Autodesk Inventor part; units mm, degrees
ref_plane "YZ Plane" through (0, 0, 0) normal (1, 0, 0) x (0, 1, 0)
ref_plane "XZ Plane" through (0, 0, 0) normal (0, 1, 0) x (-1, 0, 0)
ref_plane "XY Plane" through (0, 0, 0) normal (0, 0, 1) x (1, 0, 0)
sketch "Эскиз1" plane through (0, 0, 0) normal (0, 0, 1) x (1, 0, 0)
  circle A0 centre (0.9164, -10.9801) radius 1.6008
  arc A1 (-10.5243, 2.5819) -> (-10.0836, 1.5104) centre (-11.5836, 1.5199) ccw
  arc A2 (12.3571, 0.4579) -> (11.9164, 1.5294) centre (13.4164, 1.5199) ccw
  circle A3 centre (-11.5836, 1.5199) radius 1.5
  circle A4 centre (13.4164, 1.5199) radius 1.5
  line L0 (-21.9797, -65.2227) -> (23.8125, -65.2227)
  line L1 (23.8125, -65.2227) -> (23.8125, 68.2625)
  line L2 (23.8125, 68.2625) -> (-21.9797, 68.2625)
  line L3 (-21.9797, 68.2625) -> (-21.9797, -65.2227)
  line L4 (-21.9797, -65.2227) -> (23.8125, 68.2625) construction
  line L5 (23.8125, -65.2227) -> (-21.9797, 68.2625) construction
  point P0 (0, 0)
  point P1 (-10.0836, 1.5104)
  point P2 (12.3571, 0.4579)
  point P3 (11.9164, 1.5294)
extrude "Выдавливание1" add sketch "Эскиз1" along normal blind 3
sketch "Эскиз2" plane through (0, 0, 3) normal (0, 0, 1) x (1, 0, 0)
  line L0 (23.8125, -65.2227) -> (23.8125, 68.2625)
  line L1 (23.8125, 68.2625) -> (-21.9797, 68.2625)
  line L2 (-21.9797, 68.2625) -> (-21.9797, -65.2227)
  line L3 (-21.9797, -65.2227) -> (23.8125, -65.2227)
  circle A0 centre (-11.5836, 1.5199) radius 1.5
  circle A1 centre (13.4164, 1.5199) radius 1.5
  circle A2 centre (0.9164, -10.9801) radius 1.6008
  line L4 (-11.5836, 1.5199) -> (13.4164, 1.5199)
  line L5 (0.9164, 14.0199) -> (0.9164, -10.9801)
  circle A3 centre (0.9164, 1.5199) radius 4
  point P0 (0, 0)
  dimension "d2" = 8
extrude "Выдавливание2" cut sketch "Эскиз2" against normal blind 3 contours A3 L5 L4 | L4 L5 A3 | L5 A3 L4 | L4 A3 L5
sketch "Эскиз3" plane through (0, 0, 3) normal (0, 0, 1) x (1, 0, 0)
  circle A0 centre (0.9164, 1.5199) radius 4
  line L0 (23.8125, -65.2227) -> (23.8125, 68.2625)
  line L1 (23.8125, 68.2625) -> (-21.9797, 68.2625)
  line L2 (-21.9797, 68.2625) -> (-21.9797, -65.2227)
  line L3 (-21.9797, -65.2227) -> (23.8125, -65.2227)
  circle A1 centre (-11.5836, 1.5199) radius 1.5
  circle A2 centre (13.4164, 1.5199) radius 1.5
  circle A3 centre (0.9164, -10.9801) radius 1.6008
  line L4 (0.9164, 1.5199) -> (0.9164, 18.5199)
  circle A4 centre (0.9164, 18.5199) radius 3
  point P0 (0, 0)
  dimension "d5" = 17
  dimension "d6" = 6
extrude "Выдавливание3" add sketch "Эскиз3" along normal blind 8 contours A4
sketch "Эскиз4" plane through (0, 0, 3) normal (0, 0, 1) x (1, 0, 0)
  circle A0 centre (0.9164, 18.5199) radius 3
  circle A1 centre (0.9164, 43.7699) radius 9.5
  circle A2 centre (0.9164, 43.7699) radius 13.15
  circle A3 centre (0.9164, 18.5199) radius 3
  circle A4 centre (0.9164, 1.5199) radius 4
  line L0 (23.8125, -65.2227) -> (23.8125, 68.2625)
  line L1 (23.8125, 68.2625) -> (-21.9797, 68.2625)
  line L2 (-21.9797, 68.2625) -> (-21.9797, -65.2227)
  line L3 (-21.9797, -65.2227) -> (23.8125, -65.2227)
  circle A5 centre (-11.5836, 1.5199) radius 1.5
  circle A6 centre (13.4164, 1.5199) radius 1.5
  circle A7 centre (0.9164, -10.9801) radius 1.6008
  point P0 (0, 0)
  dimension "d17" = 42.25
  dimension "d18" = 0
extrude "Выдавливание4" add sketch "Эскиз4" along normal blind 6 contours A2
sketch "Эскиз5" plane through (0, 0, 3) normal (0, 0, 1) x (1, 0, 0)
  circle A0 centre (0.9164, -10.9801) radius 1.6008
  circle A1 centre (13.4164, 1.5199) radius 1.5
  circle A2 centre (-11.5836, 1.5199) radius 1.5
  line L0 (23.8125, -65.2227) -> (23.8125, 68.2625)
  line L1 (23.8125, 68.2625) -> (-21.9797, 68.2625)
  line L2 (-21.9797, 68.2625) -> (-21.9797, -65.2227)
  line L3 (-21.9797, -65.2227) -> (23.8125, -65.2227)
  circle A3 centre (0.9164, 43.7699) radius 13.15
  circle A4 centre (0.9164, 1.5199) radius 4
  circle A5 centre (0.9164, 43.7699) radius 3
  point P0 (0, 0)
  dimension "d12" = 6
  dimension "d16" = 0
extrude "Выдавливание5" cut sketch "Эскиз5" against normal blind 8 contours A5
sketch "Эскиз6" plane through (0.9164, 43.7699, 3) normal (0, 0, 1) x (1, 0, 0)
  circle A0 centre (0, 0) radius 7.5
  circle A1 centre (0, 0) radius 13.15
  circle A2 centre (0, 0) radius 9.5
  point P0 (-0.9164, -43.7699)
  dimension "d19" = 15
extrude "Выдавливание6" cut sketch "Эскиз6" against normal blind 1 contours A0
ref_plane "РабПлоскость1" through (0, 0, -6) normal (0, 0, -1) x (-1, 0, 0)
sketch "Эскиз7" plane through (0, 0, -6) normal (0, 0, -1) x (-1, 0, 0)
  circle A0 centre (-0.9164, 43.7699) radius 13.15
  circle A1 centre (-0.9164, 43.7699) radius 9.5
  point P0 (0, 0)
extrude "Выдавливание7" add sketch "Эскиз7" against normal blind 6
sketch "Эскиз8" plane through (0.9164, 43.7699, 9) normal (0, 0, 1) x (1, 0, 0)
  circle A0 centre (0, 0) radius 13.15
  circle A1 centre (0, 0) radius 9.5
  point P0 (-0.9164, -43.7699)
extrude "Выдавливание8" cut sketch "Эскиз8" against normal blind 6
sketch "Эскиз9" plane through (0.9164, 43.7699, -6) normal (0, 0, -1) x (-1, 0, 0)
  circle A0 centre (0, 0) radius 13.15
  point P0 (0.9164, -43.7699)
extrude "Выдавливание9" add sketch "Эскиз9" against normal blind 3
sketch "Эскиз10" plane through (0.9164, 43.7699, -3) normal (0, 0, 1) x (1, 0, 0)
  circle A0 centre (0, 0) radius 3
  circle A1 centre (0, 0) radius 7.5
  point P0 (-0.9164, -43.7699)
extrude "Выдавливание10" cut sketch "Эскиз10" against normal blind 1
sketch "Эскиз12" plane through (0, 0, 3) normal (0, 0, 1) x (1, 0, 0)
  circle A0 centre (0.9164, 18.5199) radius 3
  circle A1 centre (0.9164, 1.5199) radius 4
  line L0 (23.8125, -65.2227) -> (23.8125, 68.2625)
  line L1 (23.8125, 68.2625) -> (-21.9797, 68.2625)
  line L2 (-21.9797, 68.2625) -> (-21.9797, -65.2227)
  line L3 (-21.9797, -65.2227) -> (23.8125, -65.2227)
  circle A2 centre (-11.5836, 1.5199) radius 1.5
  circle A3 centre (13.4164, 1.5199) radius 1.5
  circle A4 centre (0.9164, -10.9801) radius 1.6008
  circle A5 centre (0.9164, 43.7699) radius 7.5
  circle A6 centre (0.9164, 43.7699) radius 9.5
  point P0 (0, 0)
  dimension "d33" = 19
extrude "Выдавливание12" cut sketch "Эскиз12" against normal blind 6 contours A5 | A6
sketch "Эскиз13" plane through (0.9164, 43.7699, -3) normal (0, 0, 1) x (1, 0, 0)
  circle A0 centre (0, 0) radius 3
  point P0 (-0.9164, -43.7699)
extrude "Выдавливание13" cut sketch "Эскиз13" against normal through all
properties part number "пластина для редуктора"
Could you check a few things on this model? Use its own coordinates, in mm. A direction names the side the tool comes from. Coordinates: 2 decimals unless noted, no trailing zeros. Write each loop counter-clockwise with the first axis right and the second up, starting at its lowest first coordinate (ties: lowest second). Pieces come first, ordered by that corner, then holes. Notation, with made-up numbers: M 64.5,-36.5 L 87.5,-36.5 A24 cw 87.5,-18.5 Z; hole C 60,85 d11. An arc over 180 degrees is marked long. One line per question, with ' | ' between items.
1) Imagine slicing it at B-B, the plane x = 19. Write out the boundary of the cut face in (y, z), and give its area (3 significant figures).
Checks:
outline: M -65.22,0 L 68.26,0 L 68.26,3 L -65.22,3 Z | area: 400 mm²
2) Imagine slicing it at C-C, the plane z = -1.25. Write out the boundary of the cut face in (x, y), and give its area (3 significant figures).
Checks:
outline: C 0.92,43.77 d26.3; hole C 0.92,43.77 d19 | area: 260 mm²
3) Imagine slicing it at A-A, the plane x = 0.5. Give the number of separate pieces and of enclosed holes in the cut face, and give its area (3 significant figures).
Checks:
separate pieces: 4 | enclosed holes: 0 | area: 432 mm²
4) If we mould it in two halves opening along Y, with no side actions, what happens to faces 1 (the face through (0.708, -12.567, 1.479)), 2 (the face through (1, 68.262, 1)), 3 (the face through (6, 2, 0))? For each: released by +Y, released by -Y, zero draft, split by the parting line, or undercut.
Checks:
face 1: undercut | face 2: released by +Y | face 3: zero draft
5) Imagine slicing it at D-D, the plane y = 54.5. Write out the boundary of the cut face in (x, z).
Checks:
outline: M -21.98,0 L -6.69,0 L -6.69,-6 L 8.52,-6 L 8.52,0 L 23.81,0 L 23.81,3 L -21.98,3 Z
6) For pin 1 Ø5 at (x, y) = (0.92, -10.98) entering from +Z; pin 2 Ø9.5 at (x, y) = (4, 41) entering from +Z; pin 3 Ø3.5 at (x, y) = (-11.58, 1.52) entering from -Z; pin 4 Ø24 at (x, y) = (0.92, 43.77) entering from -Z, each with a flat end and sliding along its axis, tell me the tip position at first contact or that it passes through.
Checks:
pin 1: z = 3 | pin 2: z = -3 | pin 3: z = 0 | pin 4: z = -6
7) I need wall thicknesses on probe 1 along Y at (x, z) = (-10.5, 0.75); probe 2 along Z at (x, y) = (22, -45); probe 3 along X at (y, z) = (49.5, 1.5). Which ranges of each line are inside material? Lowest first, please. Write a range as [from, to].
Checks:
probe 1: [-65.22, 0.48], [2.56, 68.26] | probe 2: [0, 3] | probe 3: [-21.98, -6.66], [8.49, 23.81]
8) For faces 4 (the face through (23.812, 1, 1)), 5 (the face through (4.1, 43.9, -4)), 6 (the face through (3.767, 30.933, -3.042)), which set-ups out of +Z, -Z, +X, -X, +Y, -Y let a thin tool reach every point of the face, with its end or its side?
Checks:
face 4: +Z, -Z, +X, +Y, -Y | face 5: +Z | face 6: -Z
